Geometry check sheet. Reference: drawing and pictorial views, mm from the part's lowest x, y, z. A direction names the side the tool comes from. Round coordinates to 2 decimals unless told otherwise and drop trailing zeros. Write each loop counter-clockwise with the first axis right and the second up, starting at its lowest first coordinate (ties: lowest second). Pieces come first, ordered by that corner, then holes. Notation, with made-up numbers: M 64.25,-22.75 L 117.25,-22.75 A38 cw 117.25,15.25 Z; hole C 47,-39.75 d1. An arc over 180 degrees is marked long. One line per item, written item: value. Start each with the question number.
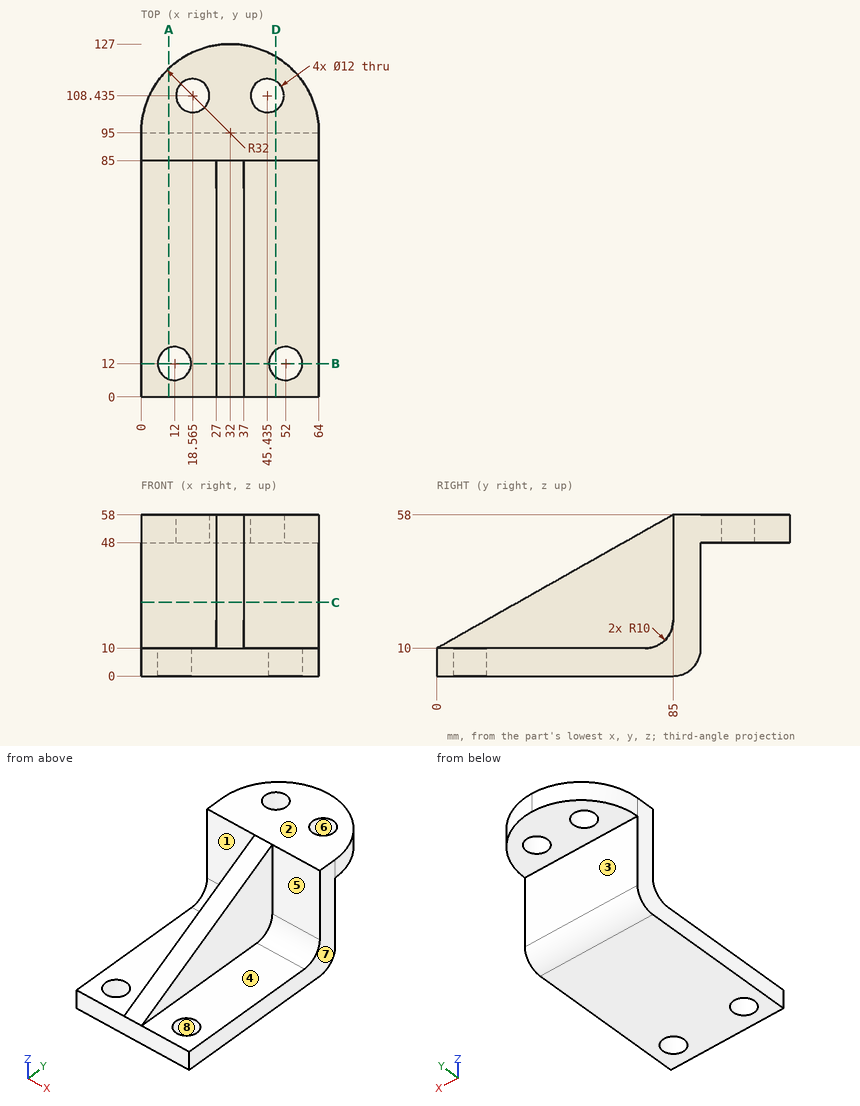
1) Gauge pin test, flat ends, axial feed: pin 1 Ø6 at (x, y) = (15.5, 51) entering from +Z; pin 2 Ø13.5 at (x, z) = (7, 31) entering from -Y; pin 3 Ø2 at (y, z) = (31.5, 22) entering from -X; pin 4 Ø9.5 at (x, y) = (45.44, 108.44) entering from +Z. Record the tip position at first contact, or that the pin passes through.
2) Access from +Z, -Z, +X, -X, +Y, -Y to the whole of each face (thin tool, end or side, straight path). Record for the marked faces 1, 2, 3 and 4.
3) Cross-section at C-C (z = 26.5). Record the boundary of the cut face in (x, y), then the cut area to 3 significant figures.
4) Thickness scan on line 1 (Y direction, x = 40, z = 41.5); line 2 (Z direction, x = 38, y = 39); line 3 (X direction, y = 72, z = 19.5). Record the ranges inside material, lowest first.
5) Cross-section at A-A (x = 10). Record the boundary of the cut face in (y, z), then the cut area to 3 significant figures.
6) Mould release check, pull along X, two halves, no side actions. Record for the marked faces 5, 6, 7 and 8: pulls with the +X half, pulls with the -X half, needs draft (parallel to the pull), parting line crosses it, or undercut.
7) Cross-section at D-D (x = 48.5). Record the boundary of the cut face in (y, z), then the cut area to 3 significant figures.
8) Cross-section at B-B (y = 12). Record the boundary of the cut face in (x, z), then the cut area to 3 significant figures.
Results below:
1. pin 1: stops at z = 10
1. pin 2: stops at y = 85
1. pin 3: stops at x = 27
1. pin 4: passes through
2. face 1: +Z, -X, -Y
2. face 2: +Z, +X, -X, +Y, -Y
2. face 3: -Z, +X, -X, +Y
2. face 4: +Z, +X, -Y
3. outline: M 0,85 L 27,85 L 27,29.22 L 37,29.22 L 37,85 L 64,85 L 64,95 L 0,95 Z
3. area: 1,200 mm²
4. line 1: y = 85 to 95
4. line 2: z = 0 to 10
4. line 3: x = 27 to 37
5. outline: M 0,0 L 6.34,0 L 6.34,10 L 0,10 Z; M 17.66,0 L 85,0 A10 ccw 95,10 L 95,48 L 118.24,48 L 118.24,58 L 85,58 L 85,20 A10 cw 75,10 L 17.66,10 Z
5. area: 1,550 mm²
6. face 5: needs draft
6. face 6: undercut
6. face 7: pulls with the +X half
6. face 8: undercut
7. outline: M 0,0 L 7.13,0 L 7.13,10 L 0,10 Z; M 16.87,0 L 85,0 A10 ccw 95,10 L 95,48 L 103.28,48 L 103.28,58 L 85,58 L 85,20 A10 cw 75,10 L 16.87,10 Z; M 113.59,48 L 122.42,48 L 122.42,58 L 113.59,58 Z
7. area: 1,500 mm²
8. outline: M 0,0 L 6,0 L 6,10 L 0,10 Z; M 18,0 L 46,0 L 46,10 L 37,10 L 37,16.78 L 27,16.78 L 27,10 L 18,10 Z; M 58,0 L 64,0 L 64,10 L 58,10 Z
8. area: 468 mm²
